The listing builds one solid part. Answer for the finished solid, in the listing's coordinates (mm). A direction names the side the tool comes from. Round coordinates to 2 decimals unless told otherwise and drop trailing zeros. Write each loop counter-clockwise with the first axis right and the second up, starting at its lowest first coordinate (ties: lowest second). Pieces come first, ordered by that corner, then holes.
(1) A cutting plane is placed at A-A, the plane z = 11.5. Give the vertices of the cut face in (x, y).
(2) For faces 1 (the face through (-6.325, 66, 13)), 2 (the face through (-10.604, 13, 2)), 3 (the face through (10.604, 13, 2)), determine the directions among +Z, -Z, +X, -X, +Y, -Y from which every point of the face is accessible in a straight line to the end or side of a thin tool.
(3) A cutting plane is placed at B-B, the plane x = 0. Give the vertices of the cut face in (y, z).
(4) Find the intervals of material crossed by probe 1 along Y at (x, z) = (-30.5, 20.75); probe 2 along X at (y, z) = (39, 7.25); probe 3 along Z at (x, y) = (9, 7.5), in increasing order.
(5) A cutting plane is placed at D-D, the plane y = 2.5. Give the vertices of the cut face in (x, z), and give its area (3 significant figures).
(6) A cutting plane is placed at C-C, the plane x = -29. Give the vertices of the cut face in (y, z), and give its area (3 significant figures).
(7) The mould has two halves that part along Y. Classify faces 4 (the face through (20, 67.543, 13)), 5 (the face through (-8, 65, 25.4)), 6 (the face through (31.704, 46, 13)), 7 (the face through (0, 25.4, 13)): +Y half, -Y half, draft (parallel to the pull), parting line (faces both ways), or undercut.
(8) Each of these flat-tipped pins is pushed along its axis until it touches: pin 1 Ø3 at (y, z) = (16.5, 1.5) entering from +X; pin 2 Ø5 at (x, z) = (-12, 11) entering from -Y; pin 3 Ø3 at (y, z) = (9.5, 2.5) entering from -X. Where does it stop, or does it pass through?
from build123d import *

# Parameters (mm, degrees)
SKETCH1_R             = 10.603707514
BOSS_EXTRUDE1_DEPTH   = 25.4
BOSS_EXTRUDE1_2_DEPTH = 25.4
BOSS_EXTRUDE3_DEPTH   = 3.47673544


with BuildPart() as part:
    # Sketch1 → Boss-Extrude1 (new body)
    with BuildSketch(Plane.XY):
        Circle(SKETCH1_R)
    extrude(amount=BOSS_EXTRUDE1_DEPTH)



with BuildPart() as body_2:
    # Sketch1 → Boss-Extrude1 2 (new body)
    with BuildSketch(Plane.XY):
        Polygon((-33.640809115, 67.542598602), (-33.640809115, 25.4), (33.640809115, 25.4), (33.640809115, 67.542598602), (6.3246, 67.542598602), (6.3246, 64.637417314), (31.70428, 64.637417314), (31.70428, 26.562817314), (-31.70428, 26.562817314), (-31.70428, 64.637417314), (-6.3246, 64.637417314), (-6.3246, 67.542598602), align=None)
    extrude(amount=BOSS_EXTRUDE1_2_DEPTH)


with BuildPart() as part_1:
    add(part.part)

    add(body_2.part)  # Boss-Extrude3 merges body 2
    # Sketch3 → Boss-Extrude3 (add)
    with BuildSketch(Plane(origin=(0, 0, 0), x_dir=(-1, 0, 0), z_dir=(0, 0, -1))):
        with BuildLine():
            Line((-10.603707514, 0), (-10.603707514, 25.4))
            Line((-10.603707514, 25.4), (10.603707514, 25.4))
            Line((10.603707514, 25.4), (10.603707514, 0))
            ThreePointArc((10.603707514, 0), (0, -10.603707514), (-10.603707514, 0))
        make_face()
    extrude(amount=-BOSS_EXTRUDE3_DEPTH)


solid = part_1.part
Solutions:
1. outline: (-33.64, 25.4) - (33.64, 25.4) - (33.64, 67.54) - (6.32, 67.54) - (6.32, 64.64) - (31.7, 64.64) - (31.7, 26.56) - (-31.7, 26.56) - (-31.7, 64.64) - (-6.32, 64.64) - (-6.32, 67.54) - (-33.64, 67.54) - close; circle Ø21.21 at (0, 0)
2. face 1: +Z, -Z, +Y
2. face 2: +Z, -Z, -X, -Y
2. face 3: +Z, -Z, +X, -Y
3. outline: (-10.6, 0) - (26.56, 0) - (26.56, 25.4) - (25.4, 25.4) - (25.4, 3.48) - (10.6, 3.48) - (10.6, 25.4) - (-10.6, 25.4) - close
4. probe 1: y = 25.4 to 26.56, 64.64 to 67.54
4. probe 2: x = -33.64 to -31.7, 31.7 to 33.64
4. probe 3: z = 0 to 3.48
5. outline: (-10.6, 0) - (10.6, 0) - (10.6, 3.48) - (10.3, 3.48) - (10.3, 25.4) - (-10.3, 25.4) - (-10.3, 3.48) - (-10.6, 3.48) - close
5. area: 526 mm2
6. outline: (25.4, 0) - (26.56, 0) - (26.56, 25.4) - (25.4, 25.4) - close; (64.64, 0) - (67.54, 0) - (67.54, 25.4) - (64.64, 25.4) - close
6. area: 103 mm2
7. face 4: +Y half
7. face 5: draft
7. face 6: undercut
7. face 7: undercut
8. pin 1: stops at x = 10.6
8. pin 2: stops at y = -4.71
8. pin 3: stops at x = -10.6
